Here's the drawing with two shaded views (mm, measured from the low corner). I have some questions. Give positions to 0.01 mm unless a question says otherwise; leave off trailing zeros. Write each loop counter-clockwise with the first axis right and the second up, starting at its lowest first coordinate (ties: lowest second). Pieces come first, ordered by that corner, then holes. Notation, with made-up numbers: (-30.75, -38.5) - (5.25, -38.5) arc R22 cw to (5.25, -7.5) - close; hole circle Ø1 at (55, -28.75). An arc over 180 degrees is marked (long way). Write item = value, one per line.
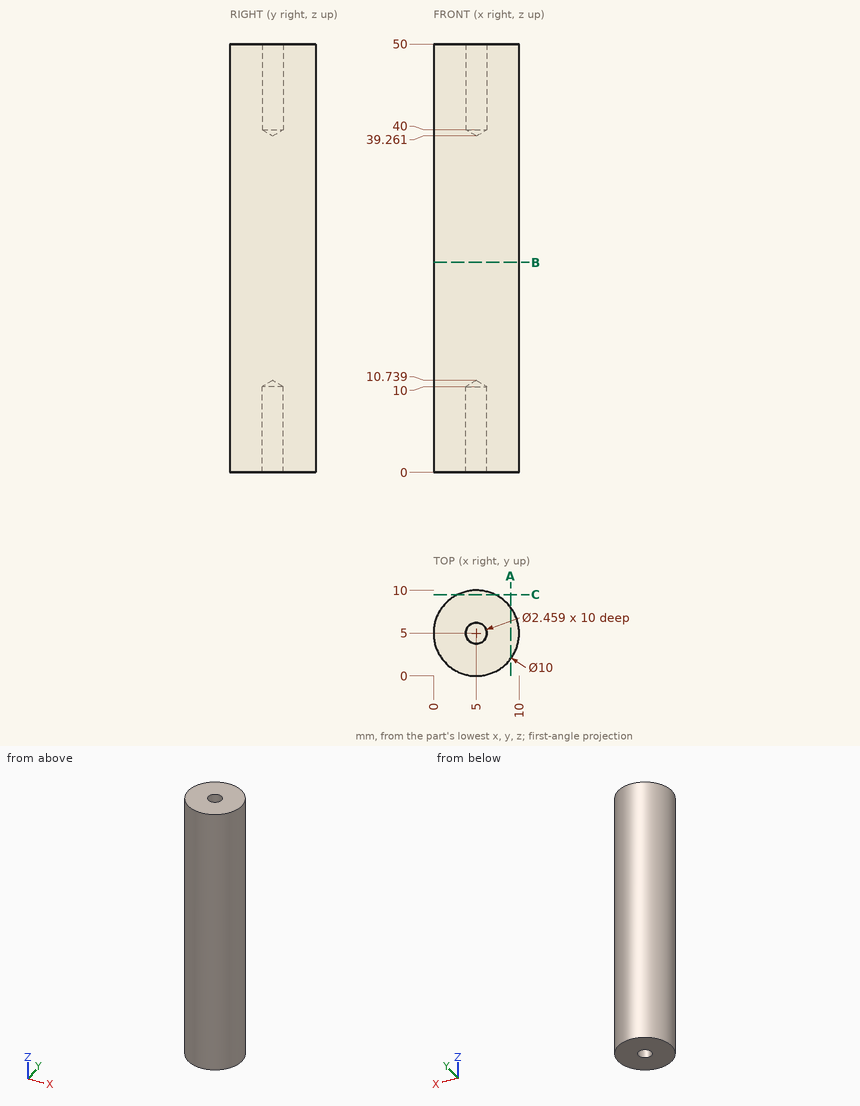
1. If we section it at C-C, the plane y = 9.5: Please give me the cut outline in (x, z).
Filled sheet:
outline = (2.82, 0) - (7.18, 0) - (7.18, 50) - (2.82, 50) - close
2. I need wall thicknesses on line 1 (Y direction, x = 5, z = 4.5); line 2 (Y direction, x = 6, z = 35). Which ranges of each line are inside material? Lowest first, please.
Filled sheet:
line_1 = 0 to 3.77, 6.23 to 10
line_2 = 0.1 to 9.9
3. For pin 1 (2 mm diameter, centred on x = 8, z = 12.5, fed in from -Y); pin 2 (1.5 mm diameter, centred on x = 8.5, z = 32, fed in from -Y); pin 3 (1.5 mm diameter, centred on x = 5, y = 5, fed in from -Z), each with a flat end and sliding along its axis, tell me the tip position at first contact or that it passes through.
Filled sheet:
pin_1 = 0.42
pin_2 = 0.82
pin_3 = 10.29
4. If we section it at A-A, the plane x = 9: Please give me the cut outline in (y, z), and give its area (3 significant figures).
Filled sheet:
outline = (2, 0) - (8, 0) - (8, 50) - (2, 50) - close
area = 300 mm2
5. If we section it at B-B, the plane z = 24.5: Please give me the cut outline in (x, y).
Filled sheet:
outline = circle Ø10 at (5, 5)
